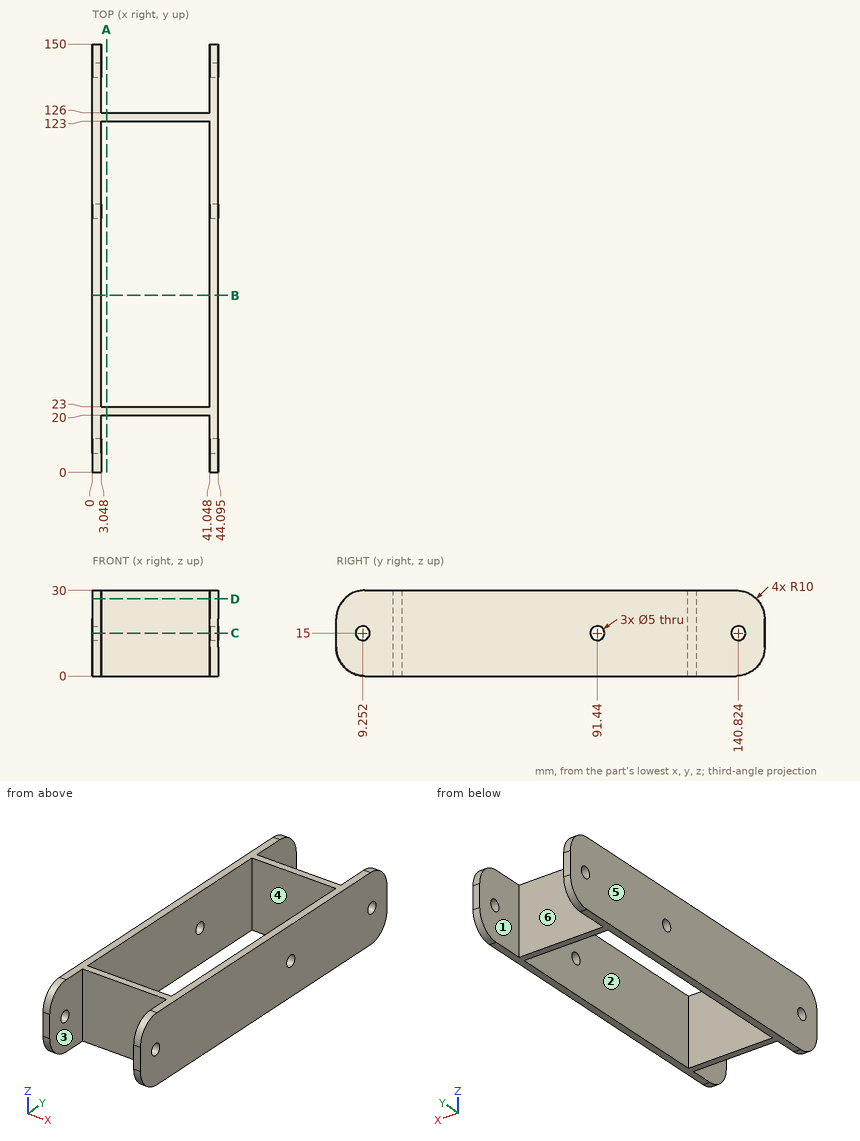
Verification items for this drawing (mm, ordinates from the low corner). A direction names the side the tool comes from. Give positions to 0.01 mm unless a question says otherwise; leave off trailing zeros. Write each loop counter-clockwise with the first axis right and the second up, starting at its lowest first coordinate (ties: lowest second). Pieces come first, ordered by that corner, then holes.
1) Section check B-B, the plane y = 62. Record the boundary of the cut face in (x, z) (1 decimal), and give its area (3 significant figures).
2) Section check C-C, the plane z = 15. State how many separate pieces and enclosed holes the cut face has, and give its area (3 significant figures).
3) Section check D-D, the plane z = 27. Record the boundary of the cut face in (x, y) (1 decimal).
4) Section check A-A, the plane x = 5. Record the boundary of the cut face in (y, z), and give its area (3 significant figures).
5) Access from +Z, -Z, +X, -X, +Y, -Y to the whole of each face (thin tool, end or side, straight path). Record for the marked faces 1, 2 and 3.
6) Gauge pin test, flat ends, axial feed: pin 1 (8 mm diameter, centred on x = 39.5, z = 4, fed in from +Y); pin 2 (6 mm diameter, centred on x = 23.5, z = 21.5, fed in from -Y); pin 3 (6 mm diameter, centred on x = 12, z = 19.5, fed in from +Y); pin 4 (10 mm diameter, centred on y = 13.5, z = 14.5, fed in from -X). Record the tip position at first contact, or that the pin passes through.
7) Release check for a two-part mould opening along Y. For the marked faces 4, 5 and 6 record: pulls with the +Y half, pulls with the -Y half, needs draft (parallel to the pull), parting line crosses it, or undercut.
8) Material ranges on L1, parallel to X at y = 33, z = 2 (1 decimal); L2, parallel to Y at x = 5, z = 18.5, recorded low to high.
Computed:
1. outline: (0, 0) - (3, 0) - (3, 30) - (0, 30) - close; (41, 0) - (44.1, 0) - (44.1, 30) - (41, 30) - close
1. area: 183 mm2
2. separate pieces: 6
2. enclosed holes: 0
2. area: 1,050 mm2
3. outline: (0, 2.9) - (3, 2.9) - (3, 20) - (41, 20) - (41, 2.9) - (44.1, 2.9) - (44.1, 147.1) - (41, 147.1) - (41, 126) - (3, 126) - (3, 147.1) - (0, 147.1) - close; hole (3, 23) - (41, 23) - (41, 123) - (3, 123) - close
4. outline: (20, 0) - (23, 0) - (23, 30) - (20, 30) - close; (123, 0) - (126, 0) - (126, 30) - (123, 30) - close
4. area: 180 mm2
5. face 1: +Z, -Z, +Y
5. face 2: +Z, -Z
5. face 3: +Z, -Z, -Y
6. pin 1: stops at y = 149.73
6. pin 2: stops at y = 20
6. pin 3: stops at y = 126
6. pin 4: stops at x = 0
7. face 4: undercut
7. face 5: needs draft
7. face 6: pulls with the +Y half
8. L1: x = 0 to 3, 41 to 44.1
8. L2: y = 20 to 23, 123 to 126
